Part print with two shaded views. Sizes in mm from the minimum x, y, z corner. A direction names the side the tool comes from. Coordinates: 2 decimals unless noted, no trailing zeros. Loops run counter-clockwise (first coordinate to the right, second up) from the corner with the lowest first, then second, coordinate; pieces in that order, holes last.
(1) Slice it at C-C (y = 13.25). Give the cut face in (x, z).
(2) Wall check: L1, parallel to Z at x = 2, y = 6.75; L2, parallel to X at y = 7, z = 24.75; L3, parallel to X at y = 9.5, z = 19. Give the ranges that are in metal, low to high.
(3) Flat gauge pins, fed straight in: P1, Ø4, axis at y = 12, z = 11, coming from the +X side (1 decimal); P2, Ø2, axis at y = 3.5, z = 7, coming from the -X side; P3, Ø1, axis at x = 10.5, z = 11, coming from the -Y side. Where does each tip first touch, or does it go through?
(4) Tool access for the marked faces 1 and 2: list every direction of +Z, -Z, +X, -X, +Y, -Y with a clear straight run to the whole face (end or side of a thin tool).
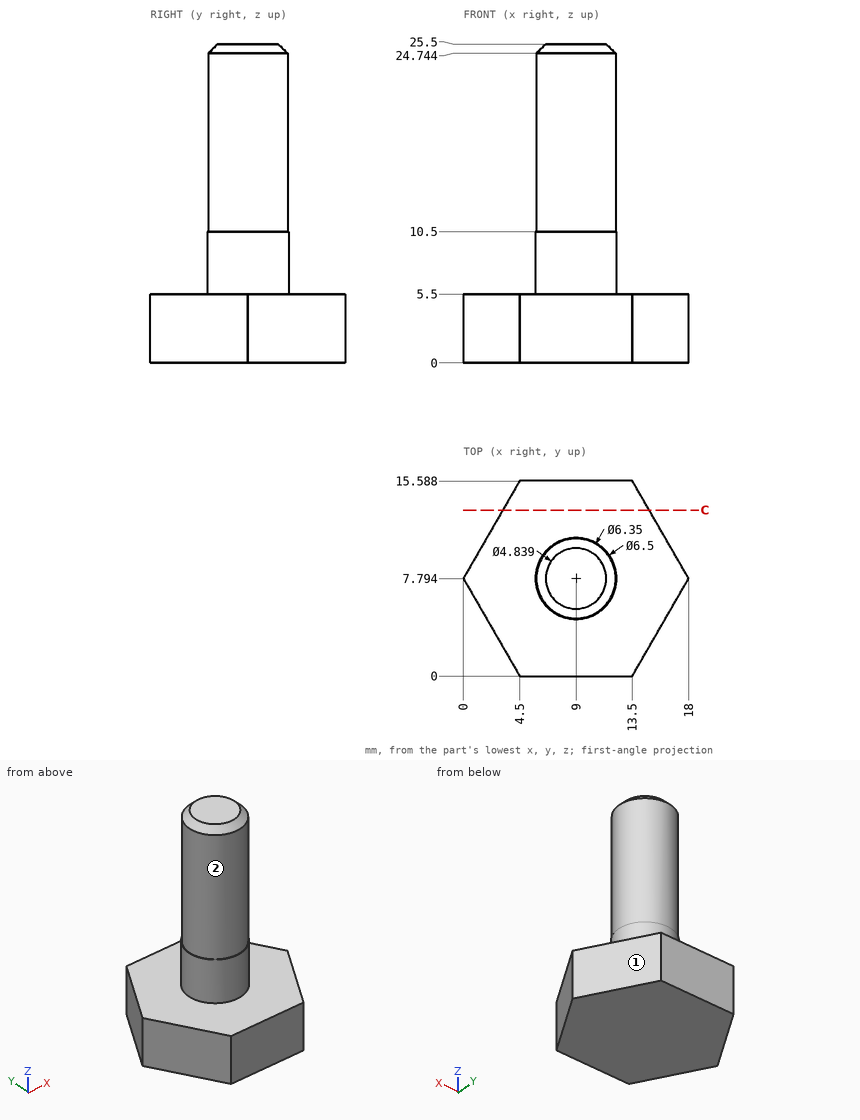
Response values:
1. outline: (3.15, 0) - (14.85, 0) - (14.85, 5.5) - (3.15, 5.5) - close
2. L1: z = 0 to 5.5
2. L2: x = 5.93 to 12.07
2. L3: x = 6.32 to 11.68
3. P1: stops at x = 11.3
3. P2: passes through
3. P3: stops at y = 4.78
4. face 1: +Z, -Z, +X, +Y
4. face 2: +Z
